The model under review builds one solid part; all positions refer to its coordinate system, in mm. Coordinates: 2 decimals unless noted, no trailing zeros. Answer as CSV lines item,"result". Start each with the question number.
from build123d import *

# Parameters (mm, degrees)
SKETCH_W            = 255
SKETCH_H            = 9
PAD_DEPTH           = 6.5
SKETCH001_R         = 1.75
POCKET_DEPTH        = 6.5
LINEARPATTERN_COUNT = 13
LINEARPATTERN_PITCH = 20


with BuildPart() as part:
    # Sketch → Pad (new body)
    with BuildSketch(Plane.XY):
        with Locations((127.5, 4.5)):
            Rectangle(SKETCH_W, SKETCH_H)
    extrude(amount=PAD_DEPTH)

    # Sketch001 (on Face6 of Pad) → Pocket (cut)
    with BuildSketch(Plane.XY.offset(6.5)):
        with Locations((7.5, 4.5)):
            Circle(SKETCH001_R)
    pocket = extrude(amount=-POCKET_DEPTH, mode=Mode.SUBTRACT)

    # LinearPattern: Pocket ×13
    with Locations(*[(i * LINEARPATTERN_PITCH, 0, 0) for i in range(1, LINEARPATTERN_COUNT)]):
        add(pocket, mode=Mode.SUBTRACT)


solid = part.part
1) Take a section at A-A on z = 1. Give the number of separate pieces and of enclosed holes in the cut face, and give its area (3 significant figures).
2) Clearance check with a flat-ended pin moving along its axis: pin 1 Ø3 at (x, y) = (187.5, 4.5) entering from +Z. State where the tip first meets the part, or that it passes through.
3) To check wall thickness, follow line 1 (Y direction, x = 107.5, z = 2.5); line 2 (Y direction, x = 126.5, z = 3.75). State the ranges of each line that lie inside material, in increasing order. Write a range as [from, to].
Results:
1,separate pieces,"1"
1,enclosed holes,"13"
1,area,"2,170 mm²"
2,pin 1,"passes through"
3,line 1,"y = [0, 2.75], [6.25, 9]"
3,line 2,"y = [0, 3.06], [5.94, 9]"
